```python
from build123d import *

# Parameters (mm, degrees)
SKETCH1_W           = 65
SKETCH1_H           = 15
BOSS_EXTRUDE1_DEPTH = 4
SKETCH2_W           = 45
SKETCH2_H           = 15
BOSS_EXTRUDE2_DEPTH = 56
SKETCH3_R           = 5
CUT_EXTRUDE1_DEPTH  = 10
CUT_EXTRUDE4_REACH  = 6
SKETCH5_R           = 1.5
CUT_EXTRUDE5_REACH  = 17


with BuildPart() as part:
    # Sketch1 → Boss-Extrude1 (new body)
    with BuildSketch(Plane(origin=(0, 0, 0), x_dir=(1, 0, 0), z_dir=(0, 1, 0))):
        Rectangle(SKETCH1_W, SKETCH1_H)
    extrude(amount=BOSS_EXTRUDE1_DEPTH)

    # Sketch2 → Boss-Extrude2 (add)
    with BuildSketch(Plane(origin=(0, 4, 0), x_dir=(1, 0, 0), z_dir=(0, 1, 0))):
        Rectangle(SKETCH2_W, SKETCH2_H)
    extrude(amount=BOSS_EXTRUDE2_DEPTH)

    # Sketch3 → Cut-Extrude1 (cut)
    with BuildSketch(Plane.XY.offset(7.5)):
        with Locations((0, 51)):
            Circle(SKETCH3_R)
    extrude(amount=-CUT_EXTRUDE1_DEPTH, mode=Mode.SUBTRACT)

    # Sketch5 → Cut-Extrude4 (cut, up to next)
    with BuildSketch(Plane(origin=(0, 4, 0), x_dir=(1, 0, 0), z_dir=(0, 1, 0)), mode=Mode.PRIVATE) as cut_extrude4_sk1:
        with Locations((-27.5, 0)):
            Circle(SKETCH5_R)
    cut_extrude4_tool1 = extrude(cut_extrude4_sk1.sketch, amount=-CUT_EXTRUDE4_REACH, mode=Mode.PRIVATE) & part.part
    add(cut_extrude4_tool1.solids().sort_by_distance((-27.5, 4, 0))[0], mode=Mode.SUBTRACT)
    # Sketch5 → Cut-Extrude4 (cut, up to next)
    with BuildSketch(Plane(origin=(0, 4, 0), x_dir=(1, 0, 0), z_dir=(0, 1, 0)), mode=Mode.PRIVATE) as cut_extrude4_sk2:
        with Locations((27.5, 0)):
            Circle(SKETCH5_R)
    cut_extrude4_tool2 = extrude(cut_extrude4_sk2.sketch, amount=-CUT_EXTRUDE4_REACH, mode=Mode.PRIVATE) & part.part
    add(cut_extrude4_tool2.solids().sort_by_distance((27.5, 4, 0))[0], mode=Mode.SUBTRACT)

    # Sketch6 → Cut-Extrude5 (cut, up to next)
    with BuildSketch(Plane.XY.offset(7.5), mode=Mode.PRIVATE) as cut_extrude5_sk1:
        with BuildLine():
            Line((5, 60), (22.5, 60))
            Line((22.5, 60), (22.5, 42.5))
            ThreePointArc((22.5, 42.5), (17.374368671, 54.874368671), (5, 60))
        make_face()
    cut_extrude5_tool1 = extrude(cut_extrude5_sk1.sketch, amount=-CUT_EXTRUDE5_REACH, mode=Mode.PRIVATE) & part.part
    add(cut_extrude5_tool1.solids().sort_by_distance((18.591061, 56.091061, 7.5))[0], mode=Mode.SUBTRACT)
    # Sketch6 → Cut-Extrude5 (cut, up to next)
    with BuildSketch(Plane.XY.offset(7.5), mode=Mode.PRIVATE) as cut_extrude5_sk2:
        with BuildLine():
            Line((-22.5, 42.5), (-22.5, 60))
            Line((-22.5, 60), (-5, 60))
            ThreePointArc((-5, 60), (-17.374368671, 54.874368671), (-22.5, 42.5))
        make_face()
    cut_extrude5_tool2 = extrude(cut_extrude5_sk2.sketch, amount=-CUT_EXTRUDE5_REACH, mode=Mode.PRIVATE) & part.part
    add(cut_extrude5_tool2.solids().sort_by_distance((-18.591061, 56.091061, 7.5))[0], mode=Mode.SUBTRACT)


solid = part.part
```
Part model, mm, in its own coordinate system. A direction names the side the tool comes from. Give positions to 0.01 mm unless a question says otherwise; leave off trailing zeros. Order: outer loops, then holes, each group sorted by start corner. A loop starts at its lowest first (then second) coordinate and runs counter-clockwise, first axis right, second up. Notation, with made-up numbers: (-25.75, -13) - (6.25, -13) arc R32 ccw to (6.25, 21) - close; hole circle Ø9 at (89, 51). An arc over 180 degrees is marked (long way). Use one line per item in the form item = value.
Item 1: Two-plate mould, pull along Y, no slides. Class faces 1 (the face through (0, 51, -2.5)), 2 (the face through (-28, 4, -2)), 3 (the face through (-32.5, 2, 0)): released by +Y, released by -Y, zero draft, split by the parting line, or undercut.
Solution:
face_1 = undercut
face_2 = released by +Y
face_3 = zero draft
Item 2: Slice it at B-B on x = -27.5. Give the cut face in (y, z).
Solution:
outline = (0, -7.5) - (4, -7.5) - (4, -1.5) - (0, -1.5) - close; (0, 1.5) - (4, 1.5) - (4, 7.5) - (0, 7.5) - close
Item 3: Pin check, flat tips, straight feed: pin 1 Ø3 at (x, z) = (26, -3.5) entering from +Y; pin 2 Ø2.5 at (x, z) = (27.5, 0) entering from -Y; pin 3 Ø3 at (x, z) = (7, 3.5) entering from +Y; pin 4 Ø2 at (y, z) = (45, 4.5) entering from +X. Stop position of each tip, or through.
Solution:
pin_1 = 4
pin_2 = through
pin_3 = 59.99
pin_4 = 22.44
Item 4: Probe probe 1 along X at (y, z) = (2.95, 0); probe 2 along Z at (x, y) = (-27.5, 0.9); probe 3 along Y at (x, z) = (0, 3.5). List the from-to ranges inside material, lowest first. Write a range as from..to.
Solution:
probe_1 = -32.5..-29, -26..26, 29..32.5
probe_2 = -7.5..-1.5, 1.5..7.5
probe_3 = 0..46, 56..60
Item 5: Slice it at D-D on x = -4. Give the cut face in (y, z), and give its area (3 significant figures).
Solution:
outline = (0, -7.5) - (60, -7.5) - (60, 7.5) - (54, 7.5) - (54, -2.5) - (48, -2.5) - (48, 7.5) - (0, 7.5) - close
area = 840 mm2
Item 6: Slice it at C-C on z = -3.25. Give the cut face in (x, y), and give its area (3 significant figures).
Solution:
outline = (-32.5, 0) - (32.5, 0) - (32.5, 4) - (22.5, 4) - (22.5, 42.5) arc R17.5 ccw to (5, 60) - (-5, 60) arc R17.5 ccw to (-22.5, 42.5) - (-22.5, 4) - (-32.5, 4) - close
area = 2,650 mm2
Item 7: Which spindle directions (+Z, -Z, +X, -X, +Y, -Y) get a long thin tool onto all of the face, cutting with end or side? Do faces 4 (the face through (0, 30, 7.5)), 5 (the face through (27, 4, -2)), 6 (the face through (26, 2, 0)), 7 (the face through (-22.5, 23, 0)), 8 (the face through (-0.651, 55.957, 2.57)). Say none if no direction does.
Solution:
face_4 = +Z, +X, -X, +Y, -Y
face_5 = +Z, -Z, +X, +Y
face_6 = +Y, -Y
face_7 = +Z, -Z, -X, +Y
face_8 = +Z
Item 8: Slice it at A-A on z = 0. Give the cut face in (x, y).
Solution:
outline = (-32.5, 0) - (-29, 0) - (-29, 4) - (-32.5, 4) - close; (-26, 0) - (26, 0) - (26, 4) - (22.5, 4) - (22.5, 42.5) arc R17.5 ccw to (5, 60) - (-5, 60) arc R17.5 ccw to (-22.5, 42.5) - (-22.5, 4) - (-26, 4) - close; (29, 0) - (32.5, 0) - (32.5, 4) - (29, 4) - close; hole circle Ø10 at (0, 51)
